Here's how the part is built. I have some questions about the finished solid (model axes, mm). A direction names the side the tool comes from. Give positions to 0.01 mm unless a question says otherwise; leave off trailing zeros. Loops run counter-clockwise (first coordinate to the right, second up) from the corner with the lowest first, then second, coordinate; pieces in that order, holes last.
Q1. Suppose I cut it at B-B (y = 87). List the corners of the cut face in (x, z) for me, and give its area (3 significant figures).
Q2. For faces 1 (the face through (413, -404.936, 25)), 2 (the face through (414, -401.761, 25)), which set-ups out of +Z, -Z, +X, -X, +Y, -Y let a thin tool reach every point of the face, with its end or its side?
Q3. Suppose I cut it at A-A (z = 25). List the corners of the cut face in (x, y) for me (3 decimals), and give its area (3 significant figures).
Q4. I'm going to push flat-ended pins straight in: P1, Ø4, axis at x = 394, z = 41, coming from the +Y side; P2, Ø5, axis at y = -199.5, z = 22, coming from the +X side; P3, Ø3, axis at x = 147.5, z = 21, coming from the +Y side. Where does each tip first touch, or does it pass through?
Q5. I need wall thicknesses on probe 1 along Y at (x, z) = (364, 30); probe 2 along X at (y, z) = (-2, 7.5); probe 3 along Y at (x, z) = (435, 6). Which ranges of each line are inside material? Lowest first, please.
Q6. Suppose I cut it at C-C (x = 135). List the corners of the cut face in (y, z) for me, and give its area (3 significant figures).
Autodesk Inventor part; units mm, degrees
ref_plane "YZ Plane" through (0, 0, 0) normal (1, 0, 0) x (0, 1, 0)
ref_plane "XZ Plane" through (0, 0, 0) normal (0, 1, 0) x (-1, 0, 0)
ref_plane "XY Plane" through (0, 0, 0) normal (0, 0, 1) x (1, 0, 0)
sketch "Sketch1" plane through (0, 0, 0) normal (0, 0, 1) x (1, 0, 0)
  arc A0 (-5.2229, -27.1112) -> (369.4271, -401.7612) centre (369.4271, -27.1112) ccw
  arc A1 (-8.3979, -27.1112) -> (369.4271, -404.9362) centre (369.4271, -27.1112) ccw
  line L0 (-5.2229, -27.1112) -> (-5.2229, 138.3204)
  line L1 (-5.2229, 138.3204) -> (-8.3979, 138.3204)
  line L2 (-8.3979, 138.3204) -> (-8.3979, -27.1112)
  line L3 (369.4271, -404.9362) -> (457.1448, -404.9362)
  line L4 (457.1448, -404.9362) -> (457.1448, -401.7612)
  line L5 (457.1448, -401.7612) -> (369.4271, -401.7612)
  line L6 (-5.2229, -27.1112) -> (-8.3979, -27.1112) construction
  point P0 (0, 0)
  dimension "d0" = 749.3
  dimension "d2" = 3.175
extrude "Extrusion1" add sketch "Sketch1" along normal blind 50.8
properties part number "Shooter Curve"
Solutions:
1. outline: (-8.4, 0) - (-5.22, 0) - (-5.22, 50.8) - (-8.4, 50.8) - close
1. area: 161 mm2
2. face 1: +Z, -Z, +X, -X, -Y
2. face 2: +Z, -Z, +X, +Y
3. outline: (-8.398, -27.111) arc R377.825 ccw to (369.427, -404.936) - (457.145, -404.936) - (457.145, -401.761) - (369.427, -401.761) arc R374.65 cw to (-5.223, -27.111) - (-5.223, 138.32) - (-8.398, 138.32) - close
3. area: 2,680 mm2
4. P1: stops at y = -401.76
4. P2: stops at x = 38.1
4. P3: stops at y = -327.85
5. probe 1: y = -404.9 to -401.72
5. probe 2: x = -8.4 to -5.22
5. probe 3: y = -404.94 to -401.76
6. outline: (-323.41, 0) - (-319.36, 0) - (-319.36, 50.8) - (-323.41, 50.8) - close
6. area: 206 mm2
